For this review, take the finished solid that the model builds, in its own axes (mm). Face numbers are marked on the shaded views. A direction names the side the tool comes from. Round coordinates to 2 decimals unless told otherwise and drop trailing zeros. Order: outer loops, then holes, each group sorted by start corner. A loop starts at its lowest first (then second) coordinate and runs counter-clockwise, first axis right, second up. Notation, with made-up numbers: (-2, 22) - (47, 22) arc R29 ccw to (47, 53) - close; hole circle Ø7 at (69, 0). An arc over 180 degrees is marked (long way). One line per item, written item: value.
Autodesk Inventor part; units mm, degrees
ref_plane "YZ Plane" through (0, 0, 0) normal (1, 0, 0) x (0, 1, 0)
ref_plane "XZ Plane" through (0, 0, 0) normal (0, 1, 0) x (-1, 0, 0)
ref_plane "XY Plane" through (0, 0, 0) normal (0, 0, 1) x (1, 0, 0)
sketch "Sketch1" plane through (0, 0, 0) normal (0, 0, 1) x (1, 0, 0)
  circle A0 centre (0, 0) radius 7.9375
  circle A1 centre (0, 0) radius 15.875 construction
  line L0 (0, 0) -> (0, 15.875) construction
  circle A2 centre (0, 12.7) radius 3.175
  circle A3 centre (-10.9985, 6.35) radius 3.175
  circle A4 centre (-10.9985, -6.35) radius 3.175
  circle A5 centre (0, -12.7) radius 3.175
  circle A6 centre (10.9985, -6.35) radius 3.175
  circle A7 centre (10.9985, 6.35) radius 3.175
  arc A8 (-11.3536, 9.5051) -> (-2.5548, 14.5851) centre (-12.7741, 22.1254) ccw
  circle A9 centre (-6.4241, 11.1269) radius 1.7526
  circle A10 centre (-12.8482, 0) radius 1.7526
  arc A11 (-13.9085, -5.08) -> (-13.9085, 5.08) centre (-25.5482, 0) ccw
  circle A12 centre (-6.4241, -11.1269) radius 1.7526
  arc A13 (-2.5548, -14.5851) -> (-11.3536, -9.5051) centre (-12.7741, -22.1254) ccw
  circle A14 centre (6.4241, -11.1269) radius 1.7526
  arc A15 (11.3536, -9.5051) -> (2.5548, -14.5851) centre (12.7741, -22.1254) ccw
  circle A16 centre (12.8482, 0) radius 1.7526
  arc A17 (13.9085, 5.08) -> (13.9085, -5.08) centre (25.5482, 0) ccw
  circle A18 centre (6.4241, 11.1269) radius 1.7526
  arc A19 (2.5548, 14.5851) -> (11.3536, 9.5051) centre (12.7741, 22.1254) ccw
  point P0 (-13.9085, 5.08)
  point P1 (-12.9691, 1.7484)
  point P2 (-12.9691, -1.7484)
  point P3 (-13.9085, -5.08)
  point P4 (-11.3536, -9.5051)
  point P5 (-7.9987, -10.3574)
  point P6 (-4.9704, -12.1058)
  point P7 (-2.5548, -14.5851)
  point P8 (2.5548, -14.5851)
  point P9 (4.9704, -12.1058)
  point P10 (7.9987, -10.3574)
  point P11 (11.3536, -9.5051)
  point P12 (13.9085, -5.08)
  point P13 (12.9691, -1.7484)
  point P14 (12.9691, 1.7484)
  point P15 (13.9085, 5.08)
  point P16 (11.3536, 9.5051)
  point P17 (7.9987, 10.3574)
  point P18 (4.9704, 12.1058)
  point P19 (2.5548, 14.5851)
  point P20 (-4.9704, 12.1058)
  point P21 (-7.9987, 10.3574)
  dimension "d1" = 31.75
  dimension "d2" = 6.35
  dimension "d0" = 15.875
  dimension "d5" = 360
  dimension "d7" = 12.7
  dimension "d8" = 3.5052
  dimension "d11" = 360
extrude "Extrusion1" add sketch "Sketch1" along normal blind 6.35 contours A2 | A2 A19 A18 A7 A17 A16 A6 A15 A14 A5 A13 A12 A4 A11 A10 A3 A8 A9 | A7 | A3 | A6 | A4 | A5
equation "\"d1\" = Brass_ID"
properties part number "Gyro Core" material "UHMW, White"
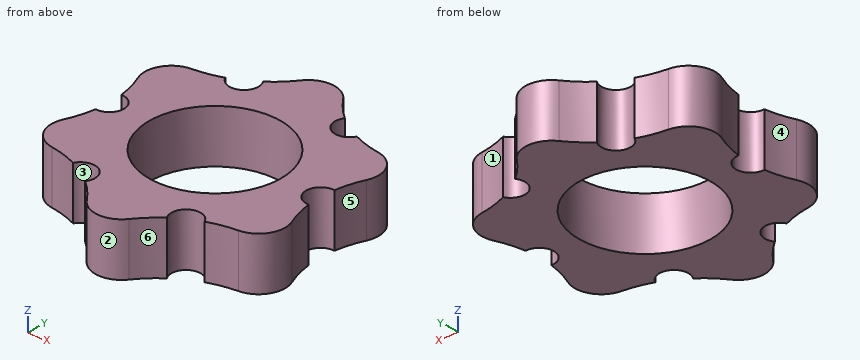
Item 1: For P1, Ø3, axis at x = 6, z = 1, coming from the -Y side; P2, Ø3, axis at x = -6, z = 3, coming from the +Y side, all flat-tipped, find the tip position at first contact; note any pin that passes through.
Returned:
P1: y = -12.49
P2: y = 12.49
Item 2: Take a section at B-B (y = 5.5). Write out the cut boundary in (x, z), plus the area to 3 significant figures.
Returned:
outline: (-14.06, 0) - (-5.72, 0) - (-5.72, 6.35) - (-14.06, 6.35) - close; (5.72, 0) - (14.06, 0) - (14.06, 6.35) - (5.72, 6.35) - close
area: 106 mm^2
Item 3: Wall thickness on line 1 (Y direction, x = 0, z = 1.75) (1 decimal); line 2 (X direction, y = -2.5, z = 2.5); line 3 (Y direction, x = 12.5, z = 0.5): over which ranges is each line inside the solid? List them lowest first.
Returned:
line 1: -15.9 to -7.9, 7.9 to 15.9
line 2: -13.1 to -7.53, 7.53 to 13.1
line 3: -9.15 to -1.72, 1.72 to 9.15
Item 4: The part is to be moulded in two halves that separate along X. For the marked faces 1, 2 and 3, say which applies: +X half, -X half, draft (parallel to the pull), parting line (faces both ways), or undercut.
Returned:
face 1: +X half
face 2: parting line
face 3: undercut
Item 5: Machinability: for the marked faces 4, 5 and 6, which of the approach directions +Z, -Z, +X, -X, +Y, -Y give a long, thin tool a straight path to every point of the face, cutting with its end or side? Answer none if there is none.
Returned:
face 4: +Z, -Z, -X
face 5: +Z, -Z, +X
face 6: +Z, -Z, +X, -Y
Item 6: Take a section at D-D (x = -10.5). Write out the cut boundary in (y, z).
Returned:
outline: (-9.63, 0) - (9.63, 0) - (9.63, 6.35) - (-9.63, 6.35) - close
